Verification items for the finished model (mm, model axes). A direction names the side the tool comes from. Round coordinates to 2 decimals unless told otherwise and drop trailing zeros. Loops run counter-clockwise (first coordinate to the right, second up) from the corner with the lowest first, then second, coordinate; pieces in that order, holes last. Notation, with made-up numbers: M 55,66.25 L 91,66.25 A20 cw 91,100.25 Z; hole C -24.5,-27.5 d6. An arc over 180 degrees is marked long. Answer as CSV lines item,"result".
```python
from build123d import *

# Parameters (mm, degrees)
F0_W      = 50.8
F0_H      = 30.48
F1_DEPTH  = 6.35
F2_R      = 1.5
F3_DEPTH  = 6.35
F4_W      = 29.2354
F4_H      = 30.48
F5_DEPTH  = 30.48
F7_DEPTH  = 30.48
F8_R      = 10.16
F9_W      = 6.35
F9_H      = 36.83
F10_DEPTH = 3.175


with BuildPart() as f1:
    # F0 (on Front) → F1 (new body)
    with BuildSketch(Plane.XZ):
        Rectangle(F0_W, F0_H)
    extrude(amount=F1_DEPTH)

    # F2 (on face) → F3 (cut, through all)
    with BuildSketch(Plane.XZ.offset(6.35)):
        with Locations((-19.05, 8.89)):
            Circle(F2_R)
        with Locations((-19.05, -8.89)):
            Circle(F2_R)
        with Locations((19.05, 8.89)):
            Circle(F2_R)
        with Locations((19.05, -8.89)):
            Circle(F2_R)
    extrude(amount=-F3_DEPTH, mode=Mode.SUBTRACT)

    # F4 (on face) → F5 (join)
    with BuildSketch(Plane.XZ.offset(6.35)):
        Rectangle(F4_W, F4_H)
    extrude(amount=F5_DEPTH)

    # F6 (on face) → F7 (cut, through all)
    with BuildSketch(Plane.XY.offset(15.24)):
        with BuildLine():
            ThreePointArc((12.7, -21.59), (8.980256, -12.609744), (0, -8.89))
            Line((0, -8.89), (0, -34.29))
            ThreePointArc((0, -34.29), (8.980256, -30.570256), (12.7, -21.59))
        make_face()
        with BuildLine():
            Line((0, -34.29), (0, -8.89))
            ThreePointArc((0, -8.89), (-12.7, -21.59), (0, -34.29))
        make_face()
    extrude(amount=-F7_DEPTH, mode=Mode.SUBTRACT)

    # F8
    f8_edges = [f1.edges().sort_by_distance(p)[0] for p in [
        (-14.6177, -36.83, 0),
        (14.6177, -36.83, 0),
    ]]
    fillet(f8_edges, radius=F8_R)

    # F9 (on face) → F10 (join)
    with BuildSketch(Plane.XY.offset(15.24)):
        with Locations((0, -18.415)):
            Rectangle(F9_W, F9_H)
    extrude(amount=-F10_DEPTH)


solid = f1.part
```
1) Draft check along Y on faces 5 (the flat face through (-3.175, -22, 14)), 6 (the flat face through (-25.4, -3, 0)), 7 (the cylindrical face through (-11.72, -33.775, 0.213)). Enter one of: +Y half, -Y half, draft (parallel to the pull), parting line (faces both ways), or undercut.
Here are the results:
face 5,"undercut"
face 6,"draft"
face 7,"-Y half"
2) Go/stop test with flat-tipped pins: pin 1 (2 mm diameter, centred on x = 15, y = -24, fed in from -Z); pin 2 (3.5 mm diameter, centred on x = 19.05, z = -8.89, fed in from -Y); pin 3 (2.5 mm diameter, centred on x = -19.05, z = 8.89, fed in from -Y); pin 4 (4 mm diameter, centred on y = -32.5, z = 4.5, fed in from -X). Record where each tip stops, or that it passes through.
Here are the results:
pin 1,"stops at z = -15.24"
pin 2,"stops at y = -6.35"
pin 3,"passes through"
pin 4,"stops at x = -13.87"
3) Section check D-D (z = -2). Record the cut outline in (x, y), plus the area to 3 significant figures.
Here are the results:
outline,"M -25.4,-6.35 L -14.62,-6.35 L -14.62,-26.67 A10.16 ccw -4.46,-36.83 L 4.46,-36.83 A10.16 ccw 14.62,-26.67 L 14.62,-6.35 L 25.4,-6.35 L 25.4,0 L -25.4,0 Z; hole C 0,-21.59 d25.4"
area,"663 mm^2"
4) Section check C-C (y = -3). Record the cut outline in (x, z).
Here are the results:
outline,"M -25.4,-15.24 L 25.4,-15.24 L 25.4,15.24 L -25.4,15.24 Z; hole C -19.05,-8.89 d3; hole C -19.05,8.89 d3; hole C 19.05,-8.89 d3; hole C 19.05,8.89 d3"
5) Section check B-B (x = 19.05). Record the cut outline in (y, z), plus the area to 3 significant figures.
Here are the results:
outline,"M -6.35,-15.24 L 0,-15.24 L 0,-10.39 L -6.35,-10.39 Z; M -6.35,-7.39 L 0,-7.39 L 0,7.39 L -6.35,7.39 Z; M -6.35,10.39 L 0,10.39 L 0,15.24 L -6.35,15.24 Z"
area,"155 mm^2"
6) Material ranges on probe 1 along Z at (x, y) = (19, -3); probe 2 along Y at (x, z) = (0, 9); probe 3 along X at (y, z) = (-3, -8), recorded low to high.
Here are the results:
probe 1,"z = -15.24 to -10.39, -7.39 to 7.39, 10.39 to 15.24"
probe 2,"y = -36.83 to -34.29, -8.89 to 0"
probe 3,"x = -25.4 to -20.26, -17.84 to 17.84, 20.26 to 25.4"
7) Set-up check for faces 1 (the flat face through (-14.618, -16, 0)), 2 (the flat face through (14.618, -16, 0)), 3 (the flat face through (3.175, -22, 14)), 4 (the flat face through (0, -21, 12.065)): record each of +Z, -Z, +X, -X, +Y, -Y from which the full face is reachable in a straight line by a thin tool's end or side.
Here are the results:
face 1,"+Z, -Z, -X, -Y"
face 2,"+Z, -Z, +X, -Y"
face 3,"+Z, -Z"
face 4,"-Z"
8) Section check A-A (z = -8.89). Record the cut outline in (x, y).
Here are the results:
outline,"M -25.4,-6.35 L -20.55,-6.35 L -20.55,0 L -25.4,0 Z; M -17.55,-6.35 L -14.62,-6.35 L -14.62,-26.67 A10.16 ccw -4.46,-36.83 L 4.46,-36.83 A10.16 ccw 14.62,-26.67 L 14.62,-6.35 L 17.55,-6.35 L 17.55,0 L -17.55,0 Z; M 20.55,-6.35 L 25.4,-6.35 L 25.4,0 L 20.55,0 Z; hole C 0,-21.59 d25.4"
